from build123d import *

# Parameters (mm, degrees)
SKETCH092_W             = 100
SKETCH092_H             = 95
PAD051_DEPTH            = 5
SKETCH115_W             = 10
SKETCH115_H             = 5
PAD071_DEPTH            = 5
LINEARPATTERN067_COUNT  = 5
LINEARPATTERN067_PITCH  = 20
SKETCH116_W             = 10
SKETCH116_H             = 5
POCKET027_DEPTH         = 5
LINEARPATTERN068_COUNT  = 5
LINEARPATTERN068_PITCH  = 20
BODY036_PLACEMENT_ANGLE = 90


with BuildPart() as part:
    # Sketch092 → Pad051 (new body)
    with BuildSketch(Plane.XY):
        Rectangle(SKETCH092_W, SKETCH092_H)
    extrude(amount=PAD051_DEPTH)

    # Sketch115 (on DatumPlane) → Pad071 (join)
    with BuildSketch(Plane(origin=(0, 47.5, 0), x_dir=(-1, 0, 0), z_dir=(0, 1, 0))):
        with Locations((-40, 2.5)):
            Rectangle(SKETCH115_W, SKETCH115_H)
    pad071 = extrude(amount=PAD071_DEPTH)

    # LinearPattern067: Pad071 ×5
    with Locations(*[(-i * LINEARPATTERN067_PITCH, 0, 0) for i in range(1, LINEARPATTERN067_COUNT)]):
        add(pad071)

    # Sketch116 (on DatumPlane) → Pocket027 (cut)
    with BuildSketch(Plane.YZ.offset(50)):
        with Locations((-37.5, 2.5)):
            Rectangle(SKETCH116_W, SKETCH116_H)
    pocket027 = extrude(amount=-POCKET027_DEPTH, mode=Mode.SUBTRACT)

    # LinearPattern068: Pocket027 ×5
    with Locations(*[(0, i * LINEARPATTERN068_PITCH, 0) for i in range(1, LINEARPATTERN068_COUNT)]):
        add(pocket027, mode=Mode.SUBTRACT)


with BuildPart() as part_1:
    # Body036 placement: moved
    add(part.part.moved(Location((55, -97.5, 55))).rotate(Axis((55, -97.5, 55), (0, -1, 0)), BODY036_PLACEMENT_ANGLE))


solid = part_1.part
The listing builds one solid part. Answer for the finished solid, in the listing's coordinates (mm). A direction names the side the tool comes from. Coordinates: 2 decimals unless noted, no trailing zeros. Write each loop counter-clockwise with the first axis right and the second up, starting at its lowest first coordinate (ties: lowest second). Pieces come first, ordered by that corner, then holes. Notation, with made-up numbers: (55, 88) - (108, 88) arc R26 cw to (108, 127) - close; hole circle Ø5 at (-22, 33). An arc over 180 degrees is marked (long way). Put each result on its own line as item: value.
1. A tool of negligible diameter and unlimited length cuts with its end or side. For faces 1 (the face through (53, -48, 10)), 2 (the face through (53, -48, 70)), 3 (the face through (52, -95, 100)), from which of +Z, -Z, +X, -X, +Y, -Y can it reach the whole face along a straight path? Write none if from no direction.
Answer sheet:
face 1: -Z, +X, -X, +Y
face 2: +X, -X, +Y
face 3: +Z, +X, -X
2. The part is cut by section A-A on y = -112. Give the vertices of the cut face in (x, z), plus the area to 3 significant figures.
Answer sheet:
outline: (50, 5) - (55, 5) - (55, 100) - (50, 100) - close
area: 475 mm^2
3. Determine the mould class of faces 4 (the face through (52, -115, 100)), 5 (the face through (53, -145, 54)), 6 (the face through (53, -48, 90)) for opening direction Y: pulls with the +Y half, pulls with the -Y half, needs draft (parallel to the pull), parting line crosses it, or undercut.
Answer sheet:
face 4: undercut
face 5: pulls with the -Y half
face 6: needs draft
4. Flat-ended cylindrical pins translate along their axes: pin 1 Ø2.5 at (x, y) = (53, -95) entering from +Z; pin 2 Ø1.5 at (x, z) = (53.5, 64) entering from +Y; pin 3 Ø1.5 at (x, z) = (51.5, 101.5) entering from +Y. Find the tip coordinate at first contact, or state that the pin passes through.
Answer sheet:
pin 1: stops at z = 100
pin 2: stops at y = -50
pin 3: stops at y = -60
5. Find the intervals of material crossed by line 1 along Z through (x, y) = (54.15, -96.5); line 2 along Y through (x, z) = (50.45, 47.5), in increasing order. Write a range as from..to.
Answer sheet:
line 1: z = 5..100
line 2: y = -145..-50
